Part print with two shaded views. Sizes in mm from the minimum x, y, z corner. A direction names the side the tool comes from. Round coordinates to 2 decimals unless told otherwise and drop trailing zeros. Order: outer loops, then holes, each group sorted by start corner. A loop starts at its lowest first (then second) coordinate and runs counter-clockwise, first axis right, second up. Notation, with made-up numbers: M 5,-3.5 L 21,-3.5 A10 cw 21,13.5 Z; hole C -23.75,83 d1. An arc over 180 degrees is marked long. Answer as a JSON object with one key per item and string values.
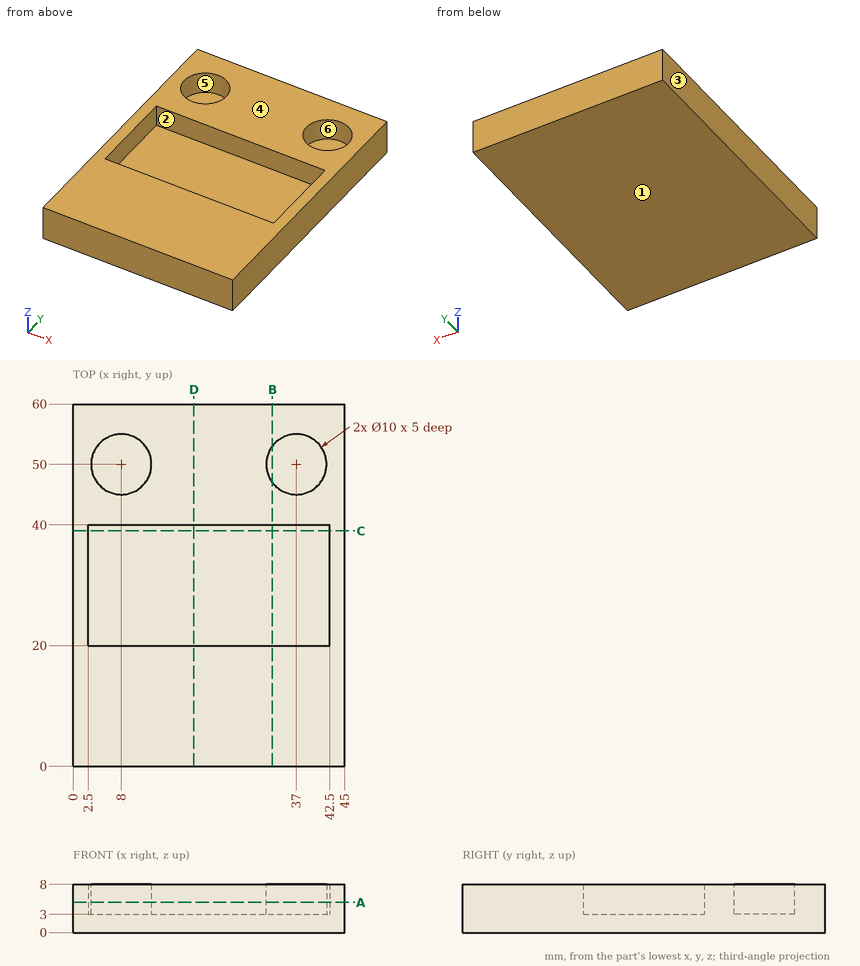
Item 1: Two-plate mould, pull along X, no slides. Class the marked faces 3, 4, 5 and 6: released by +X, released by -X, zero draft, split by the parting line, or undercut.
Worked answers:
{"face 3": "released by -X", "face 4": "zero draft", "face 5": "undercut", "face 6": "undercut"}
Item 2: Saw through at A-A on z = 5. List the corners of the cut face in (x, y).
Worked answers:
{"outline": "M 0,0 L 45,0 L 45,60 L 0,60 Z; hole M 2.5,20 L 42.5,20 L 42.5,40 L 2.5,40 Z; hole C 8,50 d10; hole C 37,50 d10"}
Item 3: Drop flat-ended pins along their axis: pin 1 Ø11.5 at (x, y) = (37, 50) entering from +Z; pin 2 Ø6 at (x, y) = (15, 26.5) entering from +Z. Give the stop position or say it passes through.
Worked answers:
{"pin 1": "stops at z = 8", "pin 2": "stops at z = 3"}
Item 4: Wall check: line 1 along Y through (x, z) = (8, 5.1); line 2 along Y through (x, z) = (25, 3.5); line 3 along Y through (x, z) = (38.5, 5.5). Give the ranges that are in metal, low to high. Write a range as [from, to].
Worked answers:
{"line 1": "y = [0, 20], [40, 45], [55, 60]", "line 2": "y = [0, 20], [40, 60]", "line 3": "y = [0, 20], [40, 45.23], [54.77, 60]"}
Item 5: 3-axis set-ups, long thin cutter, end or side, ignore diameter. For the marked faces 1 and 2: which of +Z, -Z, +X, -X, +Y, -Y reach the whole face in a straight line?
Worked answers:
{"face 1": "-Z, +X, -X, +Y, -Y", "face 2": "+Z"}
Item 6: Saw through at C-C on y = 39. List the corners of the cut face in (x, z), and give its area (3 significant figures).
Worked answers:
{"outline": "M 0,0 L 45,0 L 45,8 L 42.5,8 L 42.5,3 L 2.5,3 L 2.5,8 L 0,8 Z", "area": "160 mm2"}
Item 7: Saw through at B-B on x = 33. List the corners of the cut face in (y, z), and give its area (3 significant figures).
Worked answers:
{"outline": "M 0,0 L 60,0 L 60,8 L 53,8 L 53,3 L 47,3 L 47,8 L 40,8 L 40,3 L 20,3 L 20,8 L 0,8 Z", "area": "350 mm2"}
Item 8: Saw through at D-D on x = 20. List the corners of the cut face in (y, z).
Worked answers:
{"outline": "M 0,0 L 60,0 L 60,8 L 40,8 L 40,3 L 20,3 L 20,8 L 0,8 Z"}
